from build123d import *

# Parameters (mm, degrees)
SKETCH1_W           = 174.796166906
SKETCH1_H           = 108.92723011
BOSS_EXTRUDE1_DEPTH = 43.18
SKETCH2_R           = 7.697413188
SKETCH2_R_2         = 9.430807524
CUT_EXTRUDE1_DEPTH  = 12.7
SKETCH3_RX          = 17
SKETCH3_RY          = 10
CUT_EXTRUDE2_DEPTH  = 10
SKETCH4_R           = 5
CUT_EXTRUDE3_DEPTH  = 50


with BuildPart() as part:
    # Sketch1 → Boss-Extrude1 (new body)
    with BuildSketch(Plane(origin=(0, 0, 0), x_dir=(1, 0, 0), z_dir=(0, 1, 0))):
        Rectangle(SKETCH1_W, SKETCH1_H)
    extrude(amount=BOSS_EXTRUDE1_DEPTH)

    # Sketch2 → Cut-Extrude1 (cut)
    with BuildSketch(Plane(origin=(0, 43.18, 0), x_dir=(1, 0, 0), z_dir=(0, 1, 0))):
        with Locations(Location((-72.874036632, 36.40863105, 0), (0, 0, 270))):  # turned: the seam where the file's is
            Circle(SKETCH2_R)
        with Locations(Location((70.801263176, -36.157833353, 0), (0, 0, 270))):  # turned: the seam where the file's is
            Circle(SKETCH2_R_2)
        with BuildLine():
            Line((-50.8, 12.7), (50.8, 12.7))
            ThreePointArc((50.8, 12.7), (63.5, 0), (50.8, -12.7))
            Line((50.8, -12.7), (-50.8, -12.7))
            ThreePointArc((-50.8, -12.7), (-63.5, 0), (-50.8, 12.7))
        make_face()
    extrude(amount=-CUT_EXTRUDE1_DEPTH, mode=Mode.SUBTRACT)

    # Sketch3 → Cut-Extrude2 (cut)
    with BuildSketch(Plane(origin=(0, 43.18, 0), x_dir=(1, 0, 0), z_dir=(0, 1, 0))):
        with Locations(Location((67.398083453, 34.463615055), (0, 0, 67.693794945))):
            Ellipse(SKETCH3_RX, SKETCH3_RY)
    extrude(amount=-CUT_EXTRUDE2_DEPTH, mode=Mode.SUBTRACT)

    # Sketch4 → Cut-Extrude3 (cut)
    with BuildSketch(Plane(origin=(0, 33.18, 0), x_dir=(1, 0, 0), z_dir=(0, 1, 0))):
        with Locations(Location((67.398083453, 34.463615055, 0), (0, 0, 270))):  # turned: the seam where the file's is
            Circle(SKETCH4_R)
    extrude(amount=-CUT_EXTRUDE3_DEPTH, mode=Mode.SUBTRACT)


solid = part.part
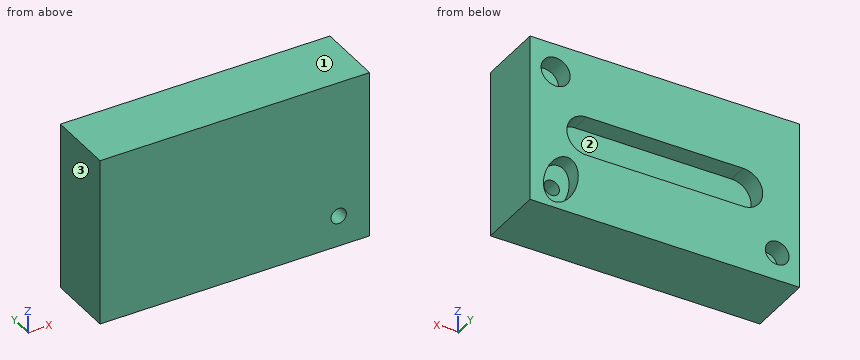
Input: part model. Units: mm. Frame: model coordinates. Face numbers are marked on the shaded views. Coordinates: 2 decimals unless noted, no trailing zeros. Loops run counter-clockwise (first coordinate to the right, second up) from the corner with the lowest first, then second, coordinate; pieces in that order, holes last. Notation, with made-up numbers: (-8, -18.75) -> (43, -18.75) arc R12 ccw to (43, 4.25) -> close; hole circle Ø5 at (69.5, 73.5). An arc over 180 degrees is marked (long way). Write item = value, one per line. Start each with the question number.
Item 1: Material intervals for line 1 (Z direction, x = 42.5, y = 41); line 2 (Y direction, x = 35, z = -11.5); line 3 (X direction, y = 35.5, z = -2.5), sorted ascending.
Item 2: First-contact query: P1, Ø8, axis at x = 67.4, z = -34.46, coming from the -Y side; P2, Ø7.5, axis at x = -75.5, z = -39, coming from the +Y side; P3, Ø20.5, axis at x = -8, z = 3, coming from the +Y side. Flat tips, straight axial feed; report the tip coordinate or a pass-through.
Item 3: Mould query, pull axis Z, two halves, no side actions, for the marked faces 1, 2 and 3. Classes: pulls with the +Z half, pulls with the -Z half, needs draft (parallel to the pull), parting line crosses it, or undercut.
Item 4: Cut plane B-B, the plane x = 4.5. Return loops of the section in (y, z), plus the area to 3 significant figures.
Item 5: Cut plane A-A, the plane z = 0. Return loops of the section in (x, y).
Ans:
q1.line_1 = -54.46 to -12.7, 12.7 to 54.46
q1.line_2 = 0 to 30.48
q1.line_3 = -87.4 to -63.25, 63.25 to 87.4
q2.P1 = through
q2.P2 = 30.48
q2.P3 = 43.18
q3.face_1 = pulls with the +Z half
q3.face_2 = undercut
q3.face_3 = needs draft
q4.outline = (0, -54.46) -> (43.18, -54.46) -> (43.18, -12.7) -> (30.48, -12.7) -> (30.48, 12.7) -> (43.18, 12.7) -> (43.18, 54.46) -> (0, 54.46) -> close
q4.area = 4,380 mm²
q5.outline = (-87.4, 0) -> (87.4, 0) -> (87.4, 43.18) -> (63.5, 43.18) -> (63.5, 30.48) -> (-63.5, 30.48) -> (-63.5, 43.18) -> (-87.4, 43.18) -> close
